from build123d import *

# Parameters (mm, degrees)
CROQUIS1_W                = 115
CROQUIS1_H                = 70
SALIENTE_EXTRUIR1_DEPTH   = 1.5
CROQUIS2_W                = 19.166666667
CROQUIS2_H                = 3
CROQUIS2_R                = 1.15
SALIENTE_EXTRUIR2_DEPTH   = 1.5
MATRIZL1_COUNT            = 3
MATRIZL1_PITCH            = 38.333333333
SIMETR_A1_COPY_1_SKETCH_W = 19.166666667
SIMETR_A1_COPY_1_SKETCH_H = 3
SIMETR_A1_COPY_1_SKETCH_R = 1.15
SIMETR_A1_COPY_1_DEPTH    = 1.5
SIMETR_A1_COPY_2_SKETCH_W = 19.166666667
SIMETR_A1_COPY_2_SKETCH_H = 3
SIMETR_A1_COPY_2_SKETCH_R = 1.15
SIMETR_A1_COPY_2_DEPTH    = 1.5
CORTAR_EXTRUIR1_DEPTH     = 2.5
MATRIZL2_COUNT            = 2
MATRIZL2_PITCH            = 38
SIMETR_A2_COPY_1_DEPTH    = 2.5
CROQUIS4_W                = 3
CROQUIS4_H                = 6.5
CROQUIS4_H_2              = 19
SALIENTE_EXTRUIR3_DEPTH   = 17
CROQUIS5_W                = 3
CROQUIS5_H                = 19
SALIENTE_EXTRUIR4_DEPTH   = 17


with BuildPart() as part:
    # Croquis1 → Saliente-Extruir1 (new body, symmetric)
    with BuildSketch(Plane.XY):
        Rectangle(CROQUIS1_W, CROQUIS1_H)
    extrude(amount=SALIENTE_EXTRUIR1_DEPTH, both=True)

    # Croquis2 → Saliente-Extruir2 (add, symmetric)
    with BuildSketch(Plane.XY):
        with Locations((-38.333333334, 36.5)):
            Rectangle(CROQUIS2_W, CROQUIS2_H)
        with Locations((-38.333333333, 36.5)):
            Circle(CROQUIS2_R, mode=Mode.SUBTRACT)
    saliente_extruir2 = extrude(amount=SALIENTE_EXTRUIR2_DEPTH, both=True)

    # MatrizL1: Saliente-Extruir2 ×3
    with Locations(*[(i * MATRIZL1_PITCH, 0, 0) for i in range(1, MATRIZL1_COUNT)]):
        add(saliente_extruir2)

    # Simetría1: Saliente-Extruir2 across plane
    add(saliente_extruir2.mirror(Plane.ZX))

    # Simetría1 copy 1 sketch → Simetría1 copy 1 (add, symmetric)
    with BuildSketch(Plane(origin=(38.333333333, 0, 0), x_dir=(1, 0, 0), z_dir=(0, 0, 1))):
        with Locations((-38.333333334, -36.5)):
            Rectangle(SIMETR_A1_COPY_1_SKETCH_W, SIMETR_A1_COPY_1_SKETCH_H)
        with Locations((-38.333333333, -36.5)):
            Circle(SIMETR_A1_COPY_1_SKETCH_R, mode=Mode.SUBTRACT)
    extrude(amount=SIMETR_A1_COPY_1_DEPTH, both=True)

    # Simetría1 copy 2 sketch → Simetría1 copy 2 (add, symmetric)
    with BuildSketch(Plane(origin=(76.666666667, 0, 0), x_dir=(1, 0, 0), z_dir=(0, 0, 1))):
        with Locations((-38.333333334, -36.5)):
            Rectangle(SIMETR_A1_COPY_2_SKETCH_W, SIMETR_A1_COPY_2_SKETCH_H)
        with Locations((-38.333333333, -36.5)):
            Circle(SIMETR_A1_COPY_2_SKETCH_R, mode=Mode.SUBTRACT)
    extrude(amount=SIMETR_A1_COPY_2_DEPTH, both=True)

    # Croquis3 → Cortar-Extruir1 (cut, symmetric)
    with BuildSketch(Plane.XY):
        Polygon((57.5, 28.5), (54.5, 28.5), (54.5, 20.15), (54.5, 17.85), (54.5, 9.5), (57.5, 9.5), align=None)
    cortar_extruir1 = extrude(amount=CORTAR_EXTRUIR1_DEPTH, both=True, mode=Mode.SUBTRACT)

    # MatrizL2: Cortar-Extruir1 ×2
    with Locations(*[(0, -i * MATRIZL2_PITCH, 0) for i in range(1, MATRIZL2_COUNT)]):
        add(cortar_extruir1, mode=Mode.SUBTRACT)

    # Simetría2: Cortar-Extruir1 across plane
    add(cortar_extruir1.mirror(Plane(origin=(0, 0, 0), x_dir=(0, 0, 1), z_dir=(1, 0, 0))), mode=Mode.SUBTRACT)

    # Simetría2 copy 1 sketch → Simetría2 copy 1 (cut, symmetric)
    with BuildSketch(Plane(origin=(0, -38, 0), x_dir=(-1, 0, 0), z_dir=(0, 0, 1))):
        Polygon((57.5, -28.5), (54.5, -28.5), (54.5, -20.15), (54.5, -17.85), (54.5, -9.5), (57.5, -9.5), align=None)
    extrude(amount=SIMETR_A2_COPY_1_DEPTH, both=True, mode=Mode.SUBTRACT)

    # Croquis4 → Saliente-Extruir3 (add)
    with BuildSketch(Plane.ZY.offset(57.5)):
        with Locations((0, -31.75)):
            Rectangle(CROQUIS4_W, CROQUIS4_H)
        with Locations((0, 31.75)):
            Rectangle(CROQUIS4_W, CROQUIS4_H)
        Rectangle(CROQUIS4_W, CROQUIS4_H_2)
    extrude(amount=SALIENTE_EXTRUIR3_DEPTH)

    # Croquis5 → Saliente-Extruir4 (add)
    with BuildSketch(Plane.ZY.offset(54.5)):
        with Locations((0, -19)):
            Rectangle(CROQUIS5_W, CROQUIS5_H)
        with Locations((0, 19)):
            Rectangle(CROQUIS5_W, CROQUIS5_H)
    extrude(amount=SALIENTE_EXTRUIR4_DEPTH)


solid = part.part
Verification items for the finished model (mm, model axes). A direction names the side the tool comes from. Round coordinates to 2 decimals unless told otherwise and drop trailing zeros. Order: outer loops, then holes, each group sorted by start corner. A loop starts at its lowest first (then second) coordinate and runs counter-clockwise, first axis right, second up.
1. Access from +Z, -Z, +X, -X, +Y, -Y to the whole of each face (thin tool, end or side, straight path). Record for faces 4 (the flat face through (19, -35, 0)), 5 (the flat face through (28.75, 36, 0)), 6 (the flat face through (56, -9.5, 0)), 7 (the flat face through (47.917, -37, 0)), 8 (the flat face through (-71.5, -19, 0)).
Final values:
face 4: +Z, -Z, -Y
face 5: +Z, -Z, +Y
face 6: +Z, -Z, +X
face 7: +Z, -Z, +X, -Y
face 8: +Z, -Z, -X
2. Section check A-A on z = -0.95. State how many separate pieces and enclosed holes the cut face has, then the cut area to 3 significant figures.
Final values:
separate pieces: 1
enclosed holes: 6
area: 9,330 mm2
3. Go/stop test with flat-tipped pins: P1, Ø2, axis at x = -38.33, y = -36.5, coming from the -Z side; P2, Ø1.5, axis at y = 36, z = -0.5, coming from the -X side; P3, Ø1.5, axis at x = -73.5, z = -0.5, coming from the -Y side; P4, Ø0.9, axis at y = 19, z = -0.5, coming from the +X side. Record where each tip stops, or that it passes through.
Final values:
P1: passes through
P2: stops at x = -47.92
P3: stops at y = -35
P4: stops at x = 54.5
4. Thickness scan on L1, parallel to Y at x = 0, z = 0.8; L2, parallel to Y at x = 27.5, z = -0.4; L3, parallel to X at y = 15, z = -0.9. Record the ranges inside material, lowest first.
Final values:
L1: y = -38 to -37.65, -35.35 to 35.35, 37.65 to 38
L2: y = -35 to 35
L3: x = -71.5 to 54.5
5. Section check C-C on x = -20. Record the cut outline in (y, z).
Final values:
outline: (-35, -1.5) - (35, -1.5) - (35, 1.5) - (-35, 1.5) - close
6. Section check B-B on y = 25. Record the cut outline in (x, z).
Final values:
outline: (-71.5, -1.5) - (54.5, -1.5) - (54.5, 1.5) - (-71.5, 1.5) - close
7. Release check for a two-part mould opening along X. For faces 1 (the flat face through (57.5, 0, 0)), 2 (the flat face through (-71.5, 19, 0)), 3 (the flat face through (-28.75, -36, 0)) record: +X half, -X half, draft (parallel to the pull), parting line (faces both ways), or undercut.
Final values:
face 1: +X half
face 2: -X half
face 3: undercut
